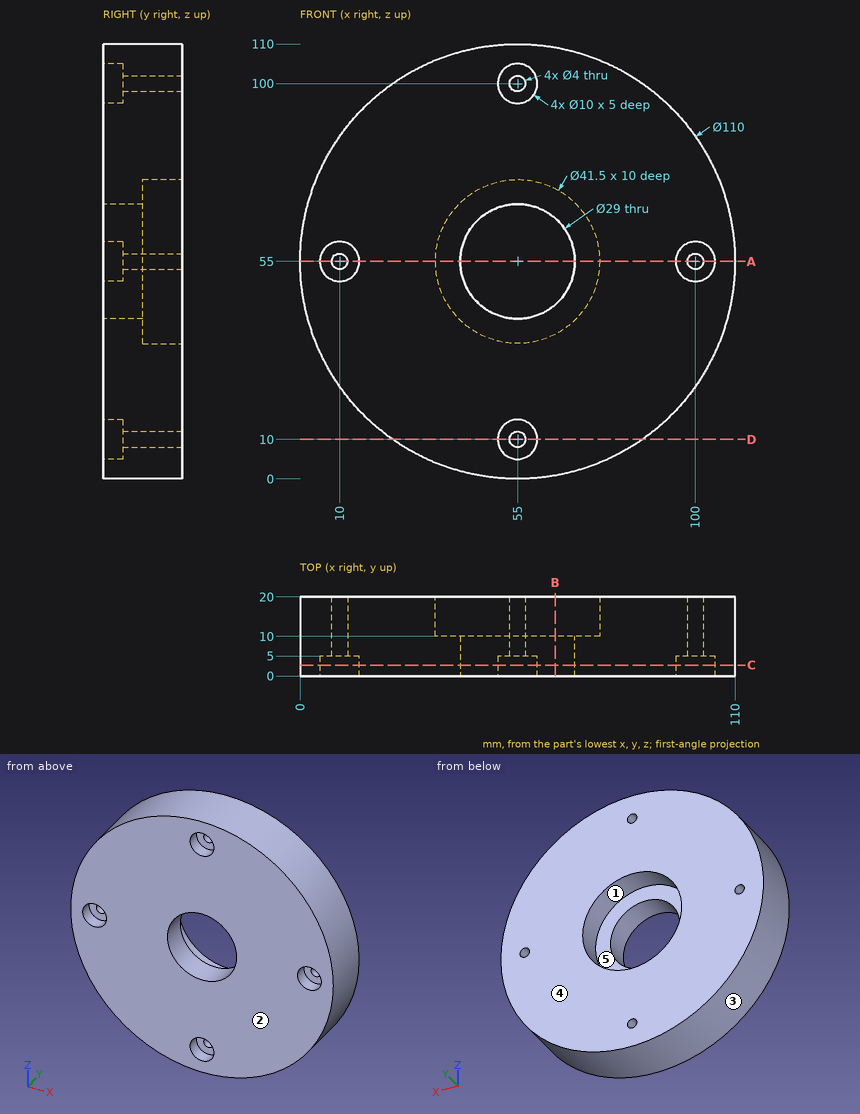
Geometry check sheet. Reference: drawing and pictorial views, mm from the part's lowest x, y, z. A direction names the side the tool comes from. Give positions to 0.01 mm unless a question says otherwise; leave off trailing zeros. Write each loop counter-clockwise with the first axis right and the second up, starting at its lowest first coordinate (ties: lowest second). Pieces come first, ordered by that corner, then holes. Notation, with made-up numbers: (-7.75, 59) - (12.25, 59) arc R29 cw to (12.25, 82) - close; hole circle Ø6 at (87, 34). An arc over 180 degrees is marked (long way). Use a Markdown table: item, result.
Q1. Go/stop test with flat-tipped pins: P1, Ø3, axis at x = 12.5, y = 5, coming from the -Z side; P2, Ø5, axis at x = 55, z = 10, coming from the -Y side; P3, Ø10, axis at x = 48, y = 15.5, coming from the +Z side. Record where each tip stops, or that it passes through.
Computed:
| item | result |
|---|---|
| P1 | stops at z = 18.34 |
| P2 | stops at y = 5 |
| P3 | stops at z = 109.96 |
Q2. Section check D-D, the plane z = 10. Enter the section's corners in (x, y).
Computed:
| item | result |
|---|---|
| outline | (23.38, 0) - (50, 0) - (50, 5) - (53, 5) - (53, 20) - (23.38, 20) - close; (57, 5) - (60, 5) - (60, 0) - (86.62, 0) - (86.62, 20) - (57, 20) - close |
Q3. Draft check along Z on the marked faces 1, 2 and 3. Enter one of: pulls with the +Z half, pulls with the -Z half, needs draft (parallel to the pull), parting line crosses it, or undercut.
Computed:
| item | result |
|---|---|
| face 1 | undercut |
| face 2 | needs draft |
| face 3 | parting line crosses it |
Q4. Section check A-A, the plane z = 55. Enter the section's corners in (x, y).
Computed:
| item | result |
|---|---|
| outline | (0, 0) - (5, 0) - (5, 5) - (8, 5) - (8, 20) - (0, 20) - close; (12, 5) - (15, 5) - (15, 0) - (40.5, 0) - (40.5, 10) - (34.25, 10) - (34.25, 20) - (12, 20) - close; (69.5, 0) - (95, 0) - (95, 5) - (98, 5) - (98, 20) - (75.75, 20) - (75.75, 10) - (69.5, 10) - close; (102, 5) - (105, 5) - (105, 0) - (110, 0) - (110, 20) - (102, 20) - close |
Q5. Set-up check for the marked faces 4 and 5: record each of +Z, -Z, +X, -X, +Y, -Y from which the full face is reachable in a straight line by a thin tool's end or side.
Computed:
| item | result |
|---|---|
| face 4 | +Z, -Z, +X, -X, +Y |
| face 5 | +Y |
Q6. Section check C-C, the plane y = 2.75. Enter the section's corners in (x, z), then the cut area to 3 significant figures.
Computed:
| item | result |
|---|---|
| outline | circle Ø110 at (55, 55); hole circle Ø10 at (10, 55); hole circle Ø29 at (55, 55); hole circle Ø10 at (55, 10); hole circle Ø10 at (55, 100); hole circle Ø10 at (100, 55) |
| area | 8,530 mm² |
Q7. Section check B-B, the plane x = 64.5. Enter the section's corners in (y, z).
Computed:
| item | result |
|---|---|
| outline | (0, 0.83) - (20, 0.83) - (20, 36.55) - (10, 36.55) - (10, 44.05) - (0, 44.05) - close; (0, 65.95) - (10, 65.95) - (10, 73.45) - (20, 73.45) - (20, 109.17) - (0, 109.17) - close |
Q8. Thickness scan on L1, parallel to X at y = 16, z = 55; L2, parallel to X at y = 8.75, z = 55. Record the ranges inside material, lowest first. Write a range as [from, to].
Computed:
| item | result |
|---|---|
| L1 | x = [0, 8], [12, 34.25], [75.75, 98], [102, 110] |
| L2 | x = [0, 8], [12, 40.5], [69.5, 98], [102, 110] |
